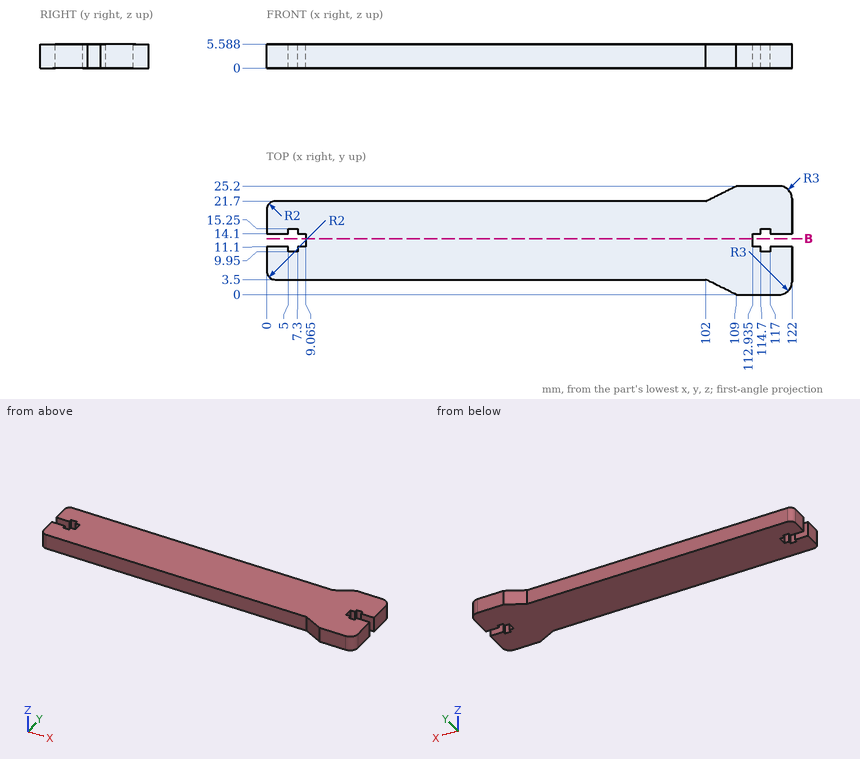
Job drawing, mm, ordinate dimensions from the low corner. One solid piece. Round coordinates to 2 decimals unless told otherwise and drop trailing zeros. Loops run counter-clockwise (first coordinate to the right, second up) from the corner with the lowest first, then second, coordinate; pieces in that order, holes last.
(1) Wall check: line 1 along X through (y, z) = (10, 4.5); line 2 along Y through (x, z) = (84, 4.7); line 3 along X through (y, z) = (20, 2.95). Give the ranges that are in metal, low to high.
(2) Cut at B-B (y = 13). Give the cut face in (x, z) (3 decimals), plus the area to 3 significant figures.
(3) Drop flat-ended pins along their axis: pin 1 (3 mm diameter, centred on x = 48.5, z = 3.5, fed in from -Y); pin 2 (0.9 mm diameter, centred on y = 13.5, z = 3.5, fed in from -X) (3 decimals); pin 3 (2.5 mm diameter, centred on x = 6, z = 3.5, fed in from +Y). Give the stop position or say it passes through.
Findings below:
1. line 1: x = 0 to 5, 7.3 to 114.7, 117 to 122
1. line 2: y = 3.5 to 21.7
1. line 3: x = 0.02 to 122
2. outline: (9.065, 0) - (112.935, 0) - (112.935, 5.588) - (9.065, 5.588) - close
2. area: 580 mm2
3. pin 1: stops at y = 3.5
3. pin 2: stops at x = 9.065
3. pin 3: stops at y = 21.7
